```python
from build123d import *

# Parameters (mm, degrees)
SKETCH1_R           = 1.6
BOSS_EXTRUDE1_DEPTH = 3
BOSS_EXTRUDE2_DEPTH = 2.5


with BuildPart() as part:
    # Sketch1 → Boss-Extrude1 (new body)
    with BuildSketch(Plane.XY):
        with BuildLine():
            Line((41.5, -10.768201729), (41.5, -13.444086969))
            ThreePointArc((41.5, -13.444086969), (39.742640687, -17.686727656), (35.5, -19.444086969))
            Line((35.5, -19.444086969), (31.703672228, -19.444086969))
            ThreePointArc((31.703672228, -19.444086969), (29.790255066, -19.063484632), (28.168138322, -17.979620875))
            Line((28.168138322, -17.979620875), (17.597242638, -7.408725191))
            ThreePointArc((17.597242638, -7.408725191), (16.513378881, -5.786608447), (16.132776544, -3.873191285))
            Line((16.132776544, -3.873191285), (16.132776544, 3.984673091))
            ThreePointArc((16.132776544, 3.984673091), (16.513378881, 5.898090253), (17.597242638, 7.520206997))
            Line((17.597242638, 7.520206997), (28.056656516, 17.979620875))
            ThreePointArc((28.056656516, 17.979620875), (29.67877326, 19.063484632), (31.592190422, 19.444086969))
            Line((31.592190422, 19.444086969), (35.5, 19.444086969))
            ThreePointArc((35.5, 19.444086969), (39.742640687, 17.686727656), (41.5, 13.444086969))
            Line((41.5, 13.444086969), (41.5, 10.768201729))
            ThreePointArc((41.5, 10.768201729), (34.795831523, 0), (41.5, -10.768201729))
        make_face()
        with Locations((37, 14.944086969)):
            Circle(SKETCH1_R, mode=Mode.SUBTRACT)
        with Locations((37, -14.944086969)):
            Circle(SKETCH1_R, mode=Mode.SUBTRACT)
    extrude(amount=BOSS_EXTRUDE1_DEPTH)

    # Sketch2 → Boss-Extrude2 (add, symmetric)
    with BuildSketch(Plane(origin=(0, 0, 0), x_dir=(1, 0, 0), z_dir=(0, 1, 0))):
        with BuildLine():
            Line((32.08575566, -3), (32.08575566, -7.515745333))
            ThreePointArc((32.08575566, -7.515745333), (29.317171973, -19.366233959), (21.584586927, -28.76337527))
            Line((21.584586927, -28.76337527), (16.996844286, -28.76337527))
            ThreePointArc((16.996844286, -28.76337527), (22.302728229, -18.521432225), (24.132776544, -7.132809616))
            Line((24.132776544, -7.132809616), (24.132776544, -3))
            Line((24.132776544, -3), (32.08575566, -3))
        make_face()
    extrude(amount=BOSS_EXTRUDE2_DEPTH, both=True)


solid = part.part
```
Part model, mm, in its own coordinate system. A direction names the side the tool comes from. Coordinates: 2 decimals unless noted, no trailing zeros. Order: outer loops, then holes, each group sorted by start corner. A loop starts at its lowest first (then second) coordinate and runs counter-clockwise, first axis right, second up. Notation, with made-up numbers: (67, -4) - (83, -4) arc R14 cw to (83, 20) - close; hole circle Ø7 at (-12.75, 61). An arc over 180 degrees is marked (long way). Return JSON: item names as keys, results as strings. Group by question number.
Item 1: Cut at B-B (x = 37). List the corners of the cut face in (y, z), plus the area to 3 significant figures.
Item 2: Pin check, flat tips, straight feed: pin 1 (1.2 mm diameter, centred on y = -1, z = 5.5, fed in from -X); pin 2 (1.4 mm diameter, centred on y = 0, z = 6.5, fed in from +X); pin 3 (2 mm diameter, centred on x = 26, y = -4.5, fed in from +Z). Stop position of each tip, or through.
Item 3: Cut at D-D (z = 26). List the corners of the cut face in (x, y), plus the area to 3 significant figures.
Item 4: Pull direction Z, two halves, no side cores. Call faces 3 (the face through (19, 0, 28.763)), 4 (the face through (24.133, 0, 5)), 5 (the face through (32.086, 0, 5)): pulls with the +Z half, pulls with the -Z half, needs draft (parallel to the pull), parting line crosses it, or undercut.
Item 5: Cut at C-C (y = 2). List the corners of the cut face in (x, z), plus the area to 3 significant figures.
Item 6: Cut at A-A (x = 18.25). List the corners of the cut face in (y, z), plus the area to 3 significant figures.
Item 7: Drill centre lines: probe 1 along Y at (x, z) = (37, 0.8); probe 2 along Z at (x, y) = (28.25, 6); probe 3 along Y at (x, z) = (27.5, 19.25). Where is each one in solid material? Low to high. Write a range as from..to.
Item 8: Which spindle directions (+Z, -Z, +X, -X, +Y, -Y) get a long thin tool onto all of the face, cutting with end or side? Do faces 1 (the face through (22.25, 0.04, 18.68)), 2 (the face through (22.754, 12.677, 1.479)). Say none if no direction does.
Check values:
{
 "1": {"outline": "(-19.25, 0) - (-16.54, 0) - (-16.54, 3) - (-19.25, 3) - close; (-13.34, 0) - (-6.93, 0) - (-6.93, 3) - (-13.34, 3) - close; (6.93, 0) - (13.34, 0) - (13.34, 3) - (6.93, 3) - close; (16.54, 0) - (19.25, 0) - (19.25, 3) - (16.54, 3) - close", "area": "54.7 mm2"},
 "2": {"pin 1": "stops at x = 24.13", "pin 2": "stops at x = 32.09", "pin 3": "stops at z = 3"},
 "3": {"outline": "(18.85, -2.5) - (24.67, -2.5) - (24.67, 2.5) - (18.85, 2.5) - close", "area": "29.1 mm2"},
 "4": {"face 3": "pulls with the +Z half", "face 4": "undercut", "face 5": "needs draft"},
 "5": {"outline": "(16.13, 0) - (34.96, 0) - (34.96, 3) - (32.09, 3) - (32.09, 7.52) arc R26.75 ccw to (21.58, 28.76) - (17, 28.76) arc R36.35 cw to (24.13, 7.13) - (24.13, 3) - (16.13, 3) - close", "area": "243 mm2"},
 "6": {"outline": "(-8.06, 0) - (8.17, 0) - (8.17, 3) - (-8.06, 3) - close; (-2.5, 26.96) - (2.5, 26.96) - (2.5, 28.76) - (-2.5, 28.76) - close", "area": "57.7 mm2"},
 "7": {"probe 1": "y = -19.25..-16.54, -13.34..-6.93, 6.93..13.34, 16.54..19.25", "probe 2": "z = 0..3", "probe 3": "y = -2.5..2.5"},
 "8": {"face 1": "-X, +Y, -Y", "face 2": "+Z, -Z, -X, +Y"}
}
